from build123d import *

# Parameters (mm, degrees)
SKETCH1_W           = 3930
SKETCH1_H           = 140
BOSS_EXTRUDE1_DEPTH = 50
SKETCH2_R           = 50
CUT_EXTRUDE1_DEPTH  = 50
SKETCH3_W           = 100
SKETCH3_H           = 140
BOSS_EXTRUDE2_DEPTH = 50
SKETCH4_R           = 50
CUT_EXTRUDE2_DEPTH  = 51
SKETCH5_W           = 1450
SKETCH5_H           = 140
SKETCH5_R           = 50
BOSS_EXTRUDE3_DEPTH = 50
SKETCH6_W           = 4130
SKETCH6_H           = 140
CUT_EXTRUDE3_DEPTH  = 50


with BuildPart() as part:
    # Sketch1 → Boss-Extrude1 (new body)
    with BuildSketch(Plane.XY):
        with Locations((1965, 70)):
            Rectangle(SKETCH1_W, SKETCH1_H)
    extrude(amount=BOSS_EXTRUDE1_DEPTH)

    # Sketch2 → Cut-Extrude1 (cut)
    with BuildSketch(Plane.XY.offset(50)):
        with Locations((3930, 70)):
            Circle(SKETCH2_R)
        with Locations((0, 70)):
            Circle(SKETCH2_R)
    extrude(amount=-CUT_EXTRUDE1_DEPTH, mode=Mode.SUBTRACT)

    # Sketch3 → Boss-Extrude2 (add, through all)
    with BuildSketch(Plane(origin=(0, 0, 0), x_dir=(-1, 0, 0), z_dir=(0, 0, -1))):
        with Locations((-3980, 70)):
            Rectangle(SKETCH3_W, SKETCH3_H)
        with Locations((50, 70)):
            Rectangle(SKETCH3_W, SKETCH3_H)
    extrude(amount=-BOSS_EXTRUDE2_DEPTH)

    # Sketch4 → Cut-Extrude2 (cut, through all)
    with BuildSketch(Plane(origin=(0, 0, 0), x_dir=(-1, 0, 0), z_dir=(0, 0, -1))):
        with Locations((0, 70)):
            Circle(SKETCH4_R)
        with Locations((-3930, 70)):
            Circle(SKETCH4_R)
    extrude(amount=-CUT_EXTRUDE2_DEPTH, mode=Mode.SUBTRACT)

    # Sketch6 → Cut-Extrude3 (cut)
    with BuildSketch(Plane.XY.offset(50)):
        with Locations((1965, 70)):
            Rectangle(SKETCH6_W, SKETCH6_H)
    extrude(amount=-CUT_EXTRUDE3_DEPTH, mode=Mode.SUBTRACT)


with BuildPart() as body_2:
    # Sketch5 → Boss-Extrude3 (new body)
    with BuildSketch(Plane(origin=(0, 0, -10), x_dir=(-1, 0, 0), z_dir=(0, 0, -1))):
        with Locations((-3305, 70)):
            Rectangle(SKETCH5_W, SKETCH5_H)
        with Locations((-3930, 70)):
            Circle(SKETCH5_R, mode=Mode.SUBTRACT)
        with Locations((-2680, 70)):
            Circle(SKETCH5_R, mode=Mode.SUBTRACT)
    extrude(amount=BOSS_EXTRUDE3_DEPTH)


solid = body_2.part
Could you check a few things on this model? Use its own coordinates, in mm. Give positions to 0.01 mm unless a question says otherwise; leave off trailing zeros. Write each loop counter-clockwise with the first axis right and the second up, starting at its lowest first coordinate (ties: lowest second). Pieces come first, ordered by that corner, then holes. Notation, with made-up numbers: (34, 11) -> (54, 11) arc R33 ccw to (54, 46) -> close; hole circle Ø6 at (-19.75, 63.5). An arc over 180 degrees is marked (long way). Answer as a JSON object with one key per item and string values.
Q1. Will this pin go through, and if not, where does the flat tip stop? pin 1 Ø4 at (x, z) = (3557, -37) entering from -Y.
Taken from the geometry:
{"pin 1": "stops at y = 0"}
Q2. Suppose I cut it at C-C on z = -35.5. Write out the boundary of the cut face in (x, y), then the cut area to 3 significant figures.
Taken from the geometry:
{"outline": "(2580, 0) -> (4030, 0) -> (4030, 140) -> (2580, 140) -> close; hole circle Ø100 at (2680, 70); hole circle Ø100 at (3930, 70)", "area": "187,000 mm²"}
Q3. Please list where these lines run through material, in increasing order: L1, parallel to Y at x = 3930, z = -46; L2, parallel to X at y = 28.5, z = -17; L3, parallel to X at y = 42, z = -52.
Taken from the geometry:
{"L1": "y = 0 to 20, 120 to 140", "L2": "x = 2580 to 2652.11, 2707.89 to 3902.11, 3957.89 to 4030", "L3": "x = 2580 to 2638.58, 2721.42 to 3888.58, 3971.42 to 4030"}
Q4. Suppose I cut it at B-B on x = 2680. Write out the boundary of the cut face in (y, z), then the cut area to 3 significant figures.
Taken from the geometry:
{"outline": "(0, -60) -> (20, -60) -> (20, -10) -> (0, -10) -> close; (120, -60) -> (140, -60) -> (140, -10) -> (120, -10) -> close", "area": "2,000 mm²"}
Q5. We'd pull the mould along Y, two halves only. Please class faces 1 (the flat face through (3315, 0, -35)), 2 (the cylindrical face through (2729.95, 72.2, -34.65)), 3 (the cylindrical face through (3883.813, 50.85, -34.65)), 4 (the flat face through (2580, 69, -35)): released by +Y, released by -Y, zero draft, split by the parting line, or undercut.
Taken from the geometry:
{"face 1": "released by -Y", "face 2": "undercut", "face 3": "undercut", "face 4": "zero draft"}
Q6. Suppose I cut it at A-A on y = 70. Write out the boundary of the cut face in (x, z).
Taken from the geometry:
{"outline": "(2580, -60) -> (2630, -60) -> (2630, -10) -> (2580, -10) -> close; (2730, -60) -> (3880, -60) -> (3880, -10) -> (2730, -10) -> close; (3980, -60) -> (4030, -60) -> (4030, -10) -> (3980, -10) -> close"}
